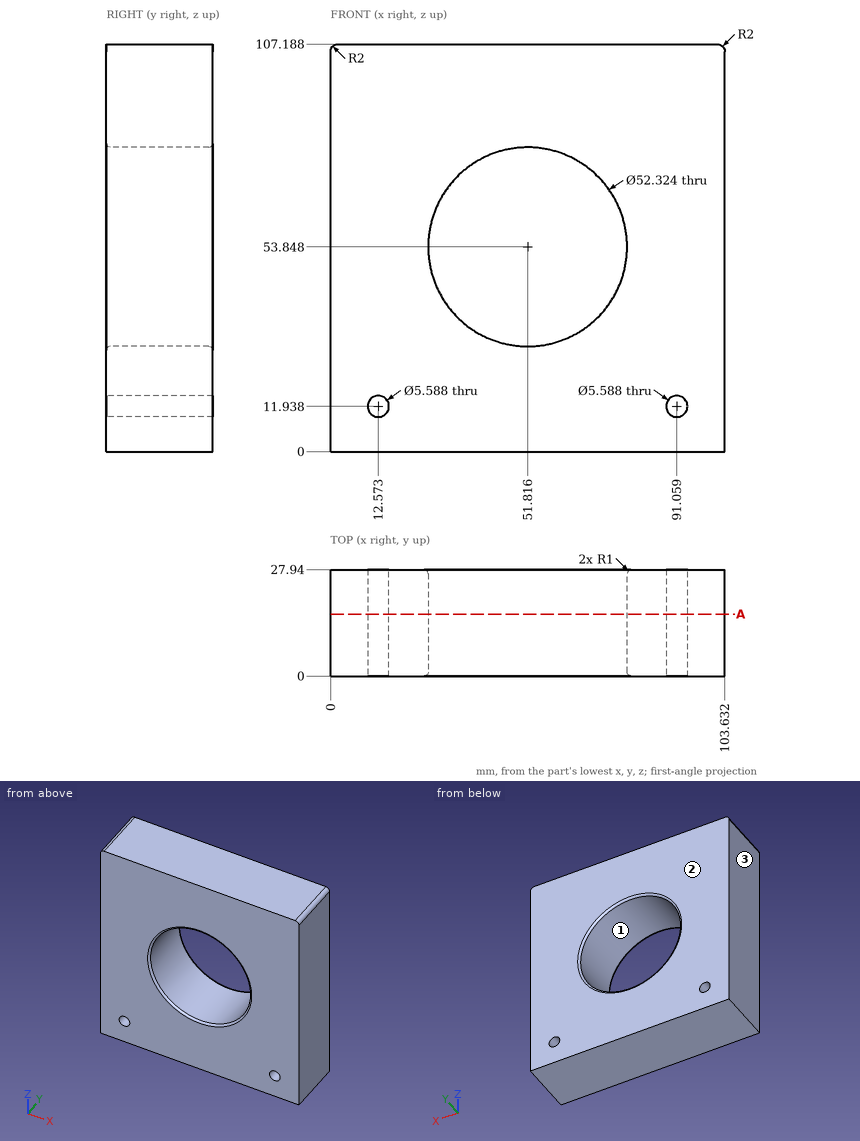
Geometry check sheet. Reference: drawing and pictorial views, mm from the part's lowest x, y, z. Round coordinates to 2 decimals unless told otherwise and drop trailing zeros. Order: outer loops, then holes, each group sorted by start corner. A loop starts at its lowest first (then second) coordinate and runs counter-clockwise, first axis right, second up. Notation, with made-up numbers: (38.25, 5) -> (42.25, 5) arc R27 cw to (42.25, 21) -> close; hole circle Ø11 at (-14, 59.25). An arc over 180 degrees is marked (long way). One line per item, written item: value. Start each with the question number.
Q1. Mould release check, pull along X, two halves, no side actions. Record for the marked faces 1, 2 and 3: pulls with the +X half, pulls with the -X half, needs draft (parallel to the pull), parting line crosses it, or undercut.
Q2. Thickness scan on line 1 (X direction, y = 22.5, z = 54); line 2 (X direction, y = 3.75, z = 49); line 3 (Z direction, x = 14.5, y = 15). Record the ranges inside material, lowest first.
Q3. Cross-section at A-A (y = 16.25). Record the boundary of the cut face in (x, z).
Completed:
1. face 1: undercut
1. face 2: needs draft
1. face 3: pulls with the -X half
2. line 1: x = 0 to 25.65, 77.98 to 103.63
2. line 2: x = 0 to 26.11, 77.52 to 103.63
2. line 3: z = 0 to 9.91, 13.96 to 107.19
3. outline: (0, 0) -> (103.63, 0) -> (103.63, 105.19) arc R2 ccw to (101.63, 107.19) -> (2, 107.19) arc R2 ccw to (0, 105.19) -> close; hole circle Ø5.59 at (12.57, 11.94); hole circle Ø52.32 at (51.82, 53.85); hole circle Ø5.59 at (91.06, 11.94)
